```python
from build123d import *

# Parameters (mm, degrees)
SKETCH2_W           = 42.3
SKETCH2_H           = 42.3
BOSS_EXTRUDE1_DEPTH = 13
SKETCH3_R           = 3
CUT_EXTRUDE1_DEPTH  = 33.613570795
SKETCH4_R           = 1.75
CUT_EXTRUDE2_DEPTH  = 33.613570795
SKETCH5_R           = 29.910616844
SKETCH5_R_2         = 27
CUT_EXTRUDE4_DEPTH  = 33.613570795
SKETCH6_R           = 3
CUT_EXTRUDE5_DEPTH  = 11
CHAMFER1_SIZE       = 1.8
SKETCH7_R           = 5.1
CUT_EXTRUDE6_DEPTH  = 1
BOSS_EXTRUDE2_START = 6
SKETCH8_R           = 16
BOSS_EXTRUDE2_DEPTH = 6
CHAMFER2_SIZE       = 1
SKETCH9_R           = 1
CUT_EXTRUDE7_DEPTH  = 3
CHAMFER3_SIZE       = 0.5


with BuildPart() as part:
    # Sketch2 → Boss-Extrude1 (new body)
    with BuildSketch(Plane(origin=(0, 0, 0), x_dir=(1, 0, 0), z_dir=(0, 1, 0))):
        Rectangle(SKETCH2_W, SKETCH2_H)
    extrude(amount=BOSS_EXTRUDE1_DEPTH)

    # Sketch3 → Cut-Extrude1 (cut, through all)
    with BuildSketch(Plane(origin=(0, 13, 0), x_dir=(1, 0, 0), z_dir=(0, 1, 0))):
        with Locations(Location((0, 0, 0), (0, 0, 270))):
            Circle(SKETCH3_R)
    extrude(amount=-CUT_EXTRUDE1_DEPTH, mode=Mode.SUBTRACT)

    # Sketch4 → Cut-Extrude2 (cut, through all)
    with BuildSketch(Plane(origin=(0, 13, 0), x_dir=(1, 0, 0), z_dir=(0, 1, 0))):
        with Locations(Location((-15.5, 15.5, 0), (0, 0, 270))):
            Circle(SKETCH4_R)
        with Locations(Location((15.5, 15.5, 0), (0, 0, 270))):
            Circle(SKETCH4_R)
        with Locations(Location((15.5, -15.5, 0), (0, 0, 270))):
            Circle(SKETCH4_R)
        with Locations(Location((-15.5, -15.5, 0), (0, 0, 270))):
            Circle(SKETCH4_R)
    extrude(amount=-CUT_EXTRUDE2_DEPTH, mode=Mode.SUBTRACT)

    # Sketch5 → Cut-Extrude4 (cut, through all)
    with BuildSketch(Plane(origin=(0, 13, 0), x_dir=(1, 0, 0), z_dir=(0, 1, 0))):
        Circle(SKETCH5_R)
        Circle(SKETCH5_R_2, mode=Mode.SUBTRACT)
    extrude(amount=-CUT_EXTRUDE4_DEPTH, mode=Mode.SUBTRACT)

    # Sketch6 → Cut-Extrude5 (cut)
    with BuildSketch(Plane(origin=(0, 13, 0), x_dir=(1, 0, 0), z_dir=(0, 1, 0))):
        with BuildLine():
            Line((-12.727922061, 12.727922061), (-21.15, 4.305844123))
            Line((-21.15, 4.305844123), (-21.15, -5.593650814))
            Line((-21.15, -5.593650814), (-17.852895433, -2.296546247))
            ThreePointArc((-17.852895433, -2.296546247), (-12.727922061, -12.727922061), (-2.296546247, -17.852895433))
            Line((-2.296546247, -17.852895433), (-5.593650814, -21.15))
            Line((-5.593650814, -21.15), (4.305844123, -21.15))
            Line((4.305844123, -21.15), (12.727922061, -12.727922061))
            ThreePointArc((12.727922061, -12.727922061), (12.727922061, 12.727922061), (-12.727922061, 12.727922061))
        make_face()
        with Locations(Location((0, 0, 0), (0, 0, 270))):
            Circle(SKETCH6_R, mode=Mode.SUBTRACT)
    extrude(amount=-CUT_EXTRUDE5_DEPTH, mode=Mode.SUBTRACT)

    # Chamfer1
    chamfer1_edges = [part.edges().sort_by_distance(p)[0] for p in [
        (-15.5, 0, 13.75),
        (15.5, 0, 13.75),
        (15.5, 0, -17.25),
        (-15.5, 0, -17.25),
    ]]
    chamfer(chamfer1_edges, length=CHAMFER1_SIZE)

    # Sketch7 → Cut-Extrude6 (cut)
    with BuildSketch(Plane(origin=(0, 2, 0), x_dir=(1, 0, 0), z_dir=(0, 1, 0))):
        with Locations(Location((0, 0, 0), (0, 0, 270))):
            Circle(SKETCH7_R)
    extrude(amount=-CUT_EXTRUDE6_DEPTH, mode=Mode.SUBTRACT)

    # Sketch8 → Boss-Extrude2 (add)
    with BuildSketch(Plane(origin=(0, 2, 0), x_dir=(1, 0, 0), z_dir=(0, 1, 0)).offset(BOSS_EXTRUDE2_START)):
        with BuildLine():
            Line((-21.15, 4.305844123), (-21.15, -5.593650814))
            Line((-21.15, -5.593650814), (-17.852895433, -2.296546247))
            ThreePointArc((-17.852895433, -2.296546247), (-12.727922061, -12.727922061), (-2.296546247, -17.852895433))
            Line((-2.296546247, -17.852895433), (-5.593650814, -21.15))
            Line((-5.593650814, -21.15), (4.305844123, -21.15))
            Line((4.305844123, -21.15), (12.727922061, -12.727922061))
            ThreePointArc((12.727922061, -12.727922061), (12.727922061, 12.727922061), (-12.727922061, 12.727922061))
            Line((-12.727922061, 12.727922061), (-21.15, 4.305844123))
        make_face()
        with Locations(Location((0, 0, 0), (0, 0, 270))):
            Circle(SKETCH8_R, mode=Mode.SUBTRACT)
    extrude(amount=-BOSS_EXTRUDE2_DEPTH)

    # Chamfer2
    chamfer2_edges = [part.edges().sort_by_distance(p)[0] for p in [
        (0, 2, -5.1),
    ]]
    chamfer(chamfer2_edges, length=CHAMFER2_SIZE - 0.0001)  # a hair under: the kernel refuses the full size

    # Sketch9 → Cut-Extrude7 (cut)
    with BuildSketch(Plane(origin=(0, 13, 0), x_dir=(1, 0, 0), z_dir=(0, 1, 0))):
        with Locations(Location((12.671572875, 18.328427125, 0), (0, 0, 270))):
            Circle(SKETCH9_R)
        with Locations(Location((18.328427125, 12.671572875, 0), (0, 0, 270))):
            Circle(SKETCH9_R)
        with Locations(Location((-12.671572875, -18.328427125, 0), (0, 0, 90))):
            Circle(SKETCH9_R)
        with Locations(Location((-18.328427125, -12.671572875, 0), (0, 0, 90))):
            Circle(SKETCH9_R)
    extrude(amount=-CUT_EXTRUDE7_DEPTH, mode=Mode.SUBTRACT)

    # Chamfer3
    chamfer3_edges = [part.edges().sort_by_distance(p)[0] for p in [
        (18.328427125, 13, -13.671572875),
        (12.671572875, 13, -19.328427125),
        (-12.671572875, 13, 19.328427125),
        (-18.328427125, 13, 13.671572875),
    ]]
    chamfer(chamfer3_edges, length=CHAMFER3_SIZE)


solid = part.part
```
Design review of the part built by this model. Coordinates are the model's own, in mm. A direction names the side the tool comes from. Coordinates: 2 decimals unless noted, no trailing zeros. Loops run counter-clockwise (first coordinate to the right, second up) from the corner with the lowest first, then second, coordinate; pieces in that order, holes last. Notation, with made-up numbers: (-32, 76.25) -> (6, 76.25) arc R20 ccw to (6, 107.25) -> close; hole circle Ø11 at (65, 16). An arc over 180 degrees is marked (long way). Answer as a JSON object with one key per item and string values.
Q1. To check wall thickness, follow L1, parallel to X at y = 0.35, z = 0; L2, parallel to X at y = 9.75, z = 15.5; L3, parallel to X at y = 10.5, z = -15.5. State the ranges of each line that lie inside material, in increasing order.
Answer block:
{"L1": "x = -21.15 to -3, 3 to 21.15", "L2": "x = -21.15 to -17.25, -13.75 to -9.15, 9.96 to 13.75, 17.25 to 21.15", "L3": "x = -21.15 to -17.25, -13.75 to -9.15, 9.15 to 13.75, 17.25 to 21.15"}
Q2. Take a section at D-D on z = -15.5. Give the boundary of the cut face in (x, y).
Answer block:
{"outline": "(-21.15, 0) -> (-19.05, 0) -> (-17.25, 1.8) -> (-17.25, 13) -> (-21.15, 13) -> close; (-13.75, 1.8) -> (-11.95, 0) -> (11.95, 0) -> (13.75, 1.8) -> (13.75, 13) -> (9.15, 13) -> (9.15, 8) -> (3.97, 8) -> (3.97, 2) -> (-3.97, 2) -> (-3.97, 8) -> (-9.15, 8) -> (-9.15, 13) -> (-13.75, 13) -> close; (17.25, 1.8) -> (19.05, 0) -> (21.15, 0) -> (21.15, 13) -> (17.25, 13) -> close"}
Q3. Tool access review of faces 5 (the flat face through (21.15, 6, 0)), 6 (the flat face through (-3.922, 10.535, 19.478)), 7 (the cylindrical face through (-18.37, 11.27, 13.67)): name each direction out of +Z, -Z, +X, -X, +Y, -Y from which nothing blocks a thin tool from reaching the whole face with its end or side.
Answer block:
{"face 5": "+Z, -Z, +X, +Y, -Y", "face 6": "+Z, +Y", "face 7": "+Y"}
Q4. Take a section at C-C on y = 3.25. Give the boundary of the cut face in (x, z).
Answer block:
{"outline": "(-21.15, -16.78) arc R27 ccw to (-16.78, -21.15) -> (16.78, -21.15) arc R27 ccw to (21.15, -16.78) -> (21.15, 16.78) arc R27 ccw to (16.78, 21.15) -> (-16.78, 21.15) arc R27 ccw to (-21.15, 16.78) -> close; hole circle Ø3.5 at (-15.5, -15.5); hole circle Ø3.5 at (-15.5, 15.5); hole circle Ø32 at (0, 0); hole circle Ø3.5 at (15.5, -15.5); hole circle Ø3.5 at (15.5, 15.5)"}
Q5. Clearance check with flat-ended pins moving along their axes: pin 1 Ø3 at (x, z) = (8.5, 8) entering from +Y; pin 2 Ø1 at (x, z) = (-18.5, 13) entering from +Y; pin 3 Ø2.5 at (x, z) = (-18.33, 12.67) entering from +Y. State where each tip first meets the part, or that it passes through.
Answer block:
{"pin 1": "stops at y = 2", "pin 2": "stops at y = 10", "pin 3": "stops at y = 12.75"}
Q6. The part is to be moulded in two halves that separate along Z. For faces 1 (the cylindrical face through (19.061, 6.591, 19.122)), 2 (the flat face through (9, 13, -16)), 3 (the cylindrical face through (0.9, 0.51, 2.86)), 4 (the cylindrical face through (-19.061, 6.591, -19.122)), say which applies: +Z half, -Z half, draft (parallel to the pull), parting line (faces both ways), or undercut.
Answer block:
{"face 1": "+Z half", "face 2": "draft", "face 3": "undercut", "face 4": "-Z half"}
